```python
from build123d import *

# Parameters (mm, degrees)
SKETCH1_W                  = 45
SKETCH1_H                  = 45
BOSS_EXTRUDE1_DEPTH        = 30
SKETCH2_R                  = 3.35
CUT_EXTRUDE1_DEPTH         = 31
SKETCH3_W                  = 4
SKETCH3_H                  = 4
PIEZOWIREFEEDTHROUGH_DEPTH = 46
ALIGNMENTHOLE_D            = 3.4544
ALIGNMENTHOLE_DEPTH        = 10
ALIGNMENTHOLE_TIP          = 1.037806461
F_0_535_40_TAPPED_HOLE1_D  = 12.7
FILLET1_R                  = 5


with BuildPart() as part:
    # Sketch1 → Boss-Extrude1 (new body)
    with BuildSketch(Plane.XY):
        with Locations((22.5, 22.5)):
            Rectangle(SKETCH1_W, SKETCH1_H)
    extrude(amount=BOSS_EXTRUDE1_DEPTH)

    # Sketch2 → Cut-Extrude1 (cut, through all)
    with BuildSketch(Plane(origin=(0, 0, 0), x_dir=(-1, 0, 0), z_dir=(0, 0, -1))):
        with Locations((-37.5, 37.5)):
            Circle(SKETCH2_R)
        with Locations((-7.5, 37.5)):
            Circle(SKETCH2_R)
        with Locations((-37.5, 7.5)):
            Circle(SKETCH2_R)
        with Locations((-7.5, 7.5)):
            Circle(SKETCH2_R)
    extrude(amount=-CUT_EXTRUDE1_DEPTH, mode=Mode.SUBTRACT)

    # Sketch3 → PiezoWireFeedthrough (cut, through all)
    with BuildSketch(Plane(origin=(45, 0, 0), x_dir=(0, 0, -1), z_dir=(1, 0, 0))):
        with Locations((-28, 22.5)):
            Rectangle(SKETCH3_W, SKETCH3_H)
    extrude(amount=-PIEZOWIREFEEDTHROUGH_DEPTH, mode=Mode.SUBTRACT)

    # AlignmentHole
    with Locations(Plane(origin=(0, 45, 0), x_dir=(1, 0, 0), z_dir=(0, 1, 0))):
        with Locations((22.5, -15)):
            Hole(ALIGNMENTHOLE_D / 2, depth=ALIGNMENTHOLE_DEPTH)
            with Locations((0, 0, -(ALIGNMENTHOLE_DEPTH + ALIGNMENTHOLE_TIP / 2))):  # 118° drill point
                Cone(0, ALIGNMENTHOLE_D / 2, ALIGNMENTHOLE_TIP, mode=Mode.SUBTRACT)

    # 0.535-40 Tapped Hole1 (through all)
    with Locations(Plane(origin=(0, 0, 0), x_dir=(-1, 0, 0), z_dir=(0, 0, -1))):
        with Locations((-22.5, 22.5)):
            Hole(F_0_535_40_TAPPED_HOLE1_D / 2)

    # Fillet1
    fillet1_edges = [part.edges().sort_by_distance(p)[0] for p in [
        (0, 45, 15),
        (45, 45, 15),
        (45, 0, 15),
        (0, 0, 15),
    ]]
    fillet(fillet1_edges, radius=FILLET1_R)


solid = part.part
```
Design review of the part built by this model. Coordinates are the model's own, in mm. A direction names the side the tool comes from. Give positions to 0.01 mm unless a question says otherwise; leave off trailing zeros. Loops run counter-clockwise (first coordinate to the right, second up) from the corner with the lowest first, then second, coordinate; pieces in that order, holes last. Notation, with made-up numbers: M -17,31.25 L -10,31.25 A16 ccw -10,60.25 Z; hole C -3.75,64.25 d3. An arc over 180 degrees is marked long. Return JSON: item names as keys, results as strings. Group by question number.
Item 1: We need section A-A (y = 37.5). Give the boundary of the cut face in (x, z), and give its area (3 significant figures).
Item 2: Mouldability with a two-part tool opening along X and no side actions: class faces 4 (the flat face through (37, 22, 26)), 5 (the cylindrical face through (10.158, 5.462, 14.79)), 6 (the cylindrical face through (35.95, 34.53, 14.79)), 7 (the flat face through (0, 22, 15)) as released by +X, released by -X, zero draft, split by the parting line, or undercut.
Item 3: We need section C-C (x = 7.5). Give the boundary of the cut face in (y, z).
Item 4: For probe 1 along Y at (x, z) = (7.5, 24); probe 2 along Y at (x, z) = (5.5, 13), list the stretches that pass through material, from the lowest coordinate up.
Item 5: Tool access review of faces 1 (the flat face through (17, 28, 0)), 2 (the flat face through (37, 20.5, 28)), 3 (the cylindrical face through (23.77, 39.93, 13.83)): name each direction out of +Z, -Z, +X, -X, +Y, -Y from which nothing blocks a thin tool from reaching the whole face with its end or side.
Item 6: We need section D-D (y = 42). Give the boundary of the cut face in (x, z).
Item 7: We need section B-B (z = 22.5). Give the boundary of the cut face in (x, y).
Item 8: Insertion check: pin 1 Ø6 at (x, y) = (37.5, 7.5) entering from -Z; pin 2 Ø16.5 at (x, y) = (22.5, 22.5) entering from -Z; pin 3 Ø1.2 at (x, y) = (40.5, 22) entering from +Z. Each pin has a flat end and moves straight along its axis. Give the tip position at first contact, or say it passes through.
Output:
{
 "1": {"outline": "M 0,0 L 4.15,0 L 4.15,30 L 0,30 Z; M 10.85,0 L 34.15,0 L 34.15,30 L 10.85,30 Z; M 40.85,0 L 45,0 L 45,30 L 40.85,30 Z; hole C 22.5,15 d3.45", "area": "939 mm^2"},
 "2": {"face 4": "zero draft", "face 5": "undercut", "face 6": "undercut", "face 7": "released by -X"},
 "3": {"outline": "M 0,0 L 4.15,0 L 4.15,30 L 0,30 Z; M 10.85,0 L 34.15,0 L 34.15,30 L 24.5,30 L 24.5,26 L 20.5,26 L 20.5,30 L 10.85,30 Z; M 40.85,0 L 45,0 L 45,30 L 40.85,30 Z"},
 "4": {"probe 1": "y = 0 to 4.15, 10.85 to 34.15, 40.85 to 45", "probe 2": "y = 0 to 4.81, 10.19 to 34.81, 40.19 to 45"},
 "5": {"face 1": "-Z, +X, -X, +Y, -Y", "face 2": "+Z, +X, -X", "face 3": "+Y"},
 "6": {"outline": "M 0.42,0 L 44.58,0 L 44.58,30 L 0.42,30 Z; hole C 22.5,15 d3.45"},
 "7": {"outline": "M 0,5 A5 ccw 5,0 L 40,0 A5 ccw 45,5 L 45,40 A5 ccw 40,45 L 5,45 A5 ccw 0,40 Z; hole C 7.5,7.5 d6.7; hole C 7.5,37.5 d6.7; hole C 22.5,22.5 d12.7; hole C 37.5,7.5 d6.7; hole C 37.5,37.5 d6.7"},
 "8": {"pin 1": "passes through", "pin 2": "stops at z = 0", "pin 3": "stops at z = 26"}
}
